from build123d import *

# Parameters (mm, degrees)
F1_DEPTH      = 40
F2_R          = 10
F3_DEPTH      = 180
F3_DEPTH_BACK = 20
F4_R          = 10
F5_DEPTH      = 20
F5_DEPTH_BACK = 180
F7_DEPTH      = 181.4
F9_DEPTH      = 244.2
F11_DEPTH     = 10
F12_R         = 2
F13_R         = 2


# Not quite as in the source:
# - a feature names something its author has since deleted; it is built from what else it names


with BuildPart() as f1:
    # F0 (on Top) → F1 (new body)
    with BuildSketch(Plane.XY):
        Polygon((-33.1370849898, -80), (33.1370849898, -80), (80, -33.1370849898), (80, 33.1370849898), (33.1370849898, 80), (-33.1370849898, 80), (-80, 33.1370849898), (-80, -33.1370849898), align=None)
        Polygon((60, -24.8528137424), (24.8528137424, -60), (-24.8528137424, -60), (-60, -24.8528137424), (-60, 24.8528137424), (-24.8528137424, 60), (24.8528137424, 60), (60, 24.8528137424), align=None, mode=Mode.SUBTRACT)
    extrude(amount=F1_DEPTH)

    # F2 (on face) → F3 (cut, two sides)
    with BuildSketch(Plane.XZ.offset(80)) as f3_sk:
        with Locations((0, 20)):
            Circle(F2_R)
    extrude(amount=-F3_DEPTH, mode=Mode.SUBTRACT)
    extrude(f3_sk.sketch, amount=F3_DEPTH_BACK, mode=Mode.SUBTRACT)

    # F4 (on face) → F5 (cut, two sides)
    with BuildSketch(Plane.YZ.offset(80)) as f5_sk:
        with Locations((0, 20)):
            Circle(F4_R)
    extrude(amount=F5_DEPTH, mode=Mode.SUBTRACT)
    extrude(f5_sk.sketch, amount=-F5_DEPTH_BACK, mode=Mode.SUBTRACT)

    # F6 (on face) → F7 (cut)
    with BuildSketch(Plane.XZ.offset(80)):
        Polygon((-33.1370849898, 40), (0, 40), (0, 51.6958795488), (-57.5, 51.6958795488), (-71.9271823764, 52.9654417948), (-71.9271823764, 40), (-57.5, 40), (-33.1370849898, 35.2627665258), align=None)
        with BuildLine():
            Line((0, 40), (0, 30))
            ThreePointArc((0, 30), (7.0710678119, 27.0710678119), (10, 20))
            Line((10, 20), (21.5, 20))
            Line((21.5, 20), (21.5, 33))
            Line((21.5, 33), (33.1370849898, 35.2627665258))
            Line((33.1370849898, 35.2627665258), (33.1370849898, 40))
            Line((33.1370849898, 40), (0, 40))
        make_face()
        Polygon((0, 51.6958795488), (0, 40), (33.1370849898, 40), (33.1370849898, 35.2627665258), (57.5, 40), (71.9271823764, 40), (71.9271823764, 52.9654417948), (57.5, 51.6958795488), align=None)
        with BuildLine():
            Line((-21.5, 20), (-10, 20))
            ThreePointArc((-10, 20), (-7.0710678119, 27.0710678119), (0, 30))
            Line((0, 30), (0, 40))
            Line((0, 40), (-33.1370849898, 40))
            Line((-33.1370849898, 40), (-33.1370849898, 35.2627665258))
            Line((-33.1370849898, 35.2627665258), (-21.5, 33))
            Line((-21.5, 33), (-21.5, 20))
        make_face()
    extrude(amount=-F7_DEPTH, mode=Mode.SUBTRACT)

    # F8 (on face) → F9 (cut)
    with BuildSketch(Plane.YZ.offset(80)):
        Polygon((33.1370849898, 0), (0, 0), (0, -11.1064584926), (57.5, -11.1064584926), (66.6687613726, -11.8878306821), (66.6687613726, 0), (57.5, 0), (33.1370849898, 4.7372334742), align=None)
        with BuildLine():
            ThreePointArc((10, 20), (7.0710678119, 12.9289321881), (0, 10))
            Line((0, 10), (0, 0))
            Line((0, 0), (33.1370849898, 0))
            Line((33.1370849898, 0), (33.1370849898, 4.7372334742))
            Line((33.1370849898, 4.7372334742), (21.5, 7))
            Line((21.5, 7), (21.5, 20))
            Line((21.5, 20), (10, 20))
        make_face()
        with BuildLine():
            ThreePointArc((0, 10), (-7.0710678119, 12.9289321881), (-10, 20))
            Line((-10, 20), (-21.5, 20))
            Line((-21.5, 20), (-21.5, 7))
            Line((-21.5, 7), (-33.1370849898, 4.7372334742))
            Line((-33.1370849898, 4.7372334742), (-33.1370849898, 0))
            Line((-33.1370849898, 0), (0, 0))
            Line((0, 0), (0, 10))
        make_face()
        Polygon((0, -11.1064584926), (0, 0), (-33.1370849898, 0), (-33.1370849898, 4.7372334742), (-57.5, 0), (-66.6687613726, 0), (-66.6687613726, -11.8878306821), (-57.5, -11.1064584926), align=None)
    extrude(amount=-F9_DEPTH, mode=Mode.SUBTRACT)

    # F10 (on face) → F11 (cut)
    with BuildSketch(Plane(origin=(56.5685424949, 56.5685424949, 0), x_dir=(-0.7071067812, 0.7071067812, 0), z_dir=(0.7071067812, 0.7071067812, 0))):
        with BuildLine():
            Line((-19.68193107, 12.9813232565), (1.7303785257, 10.0372808895))
            ThreePointArc((1.7303785257, 10.0372808895), (2.0021645777, 10.0093311061), (2.2752246058, 10))
            Line((2.2752246058, 10), (19.1370849898, 10))
            ThreePointArc((19.1370849898, 10), (21.9655121146, 11.1715728753), (23.1370849898, 14))
            Line((23.1370849898, 14), (23.1370849898, 23.055957633))
            ThreePointArc((23.1370849898, 23.055957633), (22.1519966238, 25.6847040718), (19.68193107, 27.0186767435))
            Line((19.68193107, 27.0186767435), (-1.7303785257, 29.9627191105))
            ThreePointArc((-1.7303785257, 29.9627191105), (-2.0021645777, 29.9906688939), (-2.2752246058, 30))
            Line((-2.2752246058, 30), (-19.1370849898, 30))
            ThreePointArc((-19.1370849898, 30), (-21.9655121146, 28.8284271247), (-23.1370849898, 26))
            Line((-23.1370849898, 26), (-23.1370849898, 16.944042367))
            ThreePointArc((-23.1370849898, 16.944042367), (-22.1519966238, 14.3152959282), (-19.68193107, 12.9813232565))
        make_face()
    extrude(amount=-F11_DEPTH, mode=Mode.SUBTRACT)

    # F12
    f12_edges = [f1.edges().sort_by_distance(p)[0] for p in [
        (33.137085, 65.857864, 18.527979),
        (33.965512, 65.029437, 11.171573),
        (41.92708, 57.067869, 10),
    ]]
    fillet(f12_edges, radius=F12_R)

    # F13
    f13_edges = [f1.edges().sort_by_distance(p)[0] for p in [
        (44.387085, 68.75, 0),
        (67.818542, 45.318542, 2.368617),
        (33.137085, 80, 17.631383),
        (45.318542, 67.818542, 37.631383),
        (80, 33.137085, 22.368617),
        (68.75, 44.387085, 40),
        (72.100505, 41.03658, 28.828427),
        (64.138937, 48.998148, 30),
        (57.984287, 55.152798, 29.990669),
        (50.22171, 62.915375, 28.490698),
        (40.904715, 72.23237, 25.684704),
        (40.208153, 72.928932, 18.527979),
        (41.03658, 72.100505, 11.171573),
        (48.998148, 64.138937, 10),
        (55.152798, 57.984287, 10.009331),
        (62.915375, 50.22171, 11.509302),
        (72.23237, 40.904715, 14.315296),
        (72.928932, 40.208153, 21.472021),
        (44.387085, -68.75, 0),
        (33.137085, -80, 17.631383),
        (45.318542, -67.818542, 37.631383),
        (68.75, -44.387085, 40),
        (80, -33.137085, 22.368617),
        (67.818542, -45.318542, 2.368617),
        (0, -80, 0),
        (27.318542, -80, 34.131383),
        (-44.387085, -68.75, 0),
        (-67.818542, -45.318542, 2.368617),
        (-80, -33.137085, 22.368617),
        (-68.75, -44.387085, 40),
        (-45.318542, -67.818542, 37.631383),
        (-33.137085, -80, 17.631383),
        (-44.387085, 68.75, 0),
        (-33.137085, 80, 17.631383),
        (-45.318542, 67.818542, 37.631383),
        (-68.75, 44.387085, 40),
        (-80, 33.137085, 22.368617),
        (-67.818542, 45.318542, 2.368617),
    ]]
    fillet(f13_edges, radius=F13_R)


solid = f1.part
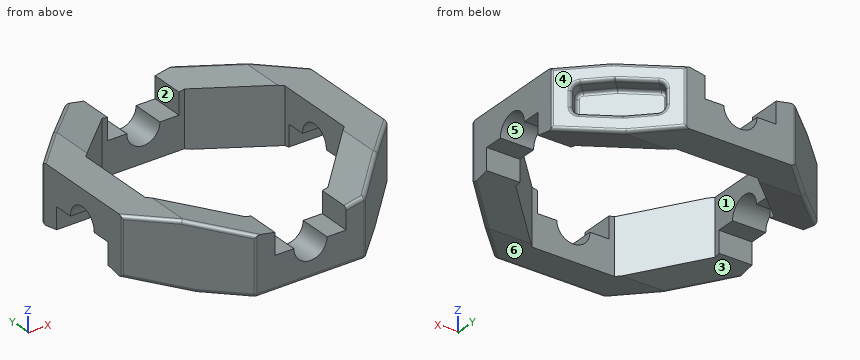
Input: part model. Units: mm. Frame: model coordinates. Face numbers are marked on the shaded views. A direction names the side the tool comes from. Round coordinates to 2 decimals unless told otherwise and drop trailing zeros. Write each loop counter-clockwise with the first axis right and the second up, starting at its lowest first coordinate (ties: lowest second). Pieces come first, ordered by that corner, then holes.
1) Ray query, L1, parallel to X at y = 36, z = 16.5; L2, parallel to Y at x = 22, z = 21. Return the intervals inside material, ascending.
2) Cut plane C-C (x = 0). Return the cut outline in (y, z).
3) Cut plane A-A (y = 0). Return the cut outline in (x, z).
4) Contact query for flat-ended pins moving along their axis: P1, Ø6.5, axis at x = 72, z = 10.5, coming from the -Y side; P2, Ø10.5, axis at y = 66, z = 25.5, coming from the +X side; P3, Ø6.5, axis at x = 69.5, z = 15.5, coming from the +Y side. Output: stop coordinate, or through.
5) Reachability of the marked faces 1, 2 and 3 from +Z, -Z, +X, -X, +Y, -Y: full face, straight path, thin tool, end or side. Return the list, or none.
6) Cut plane B-B (x = 16.5). Return the cut outline in (y, z).
7) Draft query along Y for the marked faces 4, 5 and 6. Return one class per face: pulls with the +Y half, pulls with the -Y half, needs draft (parallel to the pull), parting line crosses it, or undercut.
Geometry says:
1. L1: x = -77.14 to -48.85, 48.85 to 62.99, 68.69 to 77.14
1. L2: y = -80 to -60, 60 to 80
2. outline: (-80, 2) arc R2 ccw to (-78, 0) - (-60, 0) - (-60, 10) - (-80, 10) - close; (60, 0) - (80, 0) - (80, 10) - (60, 10) - close
3. outline: (-80, 30) - (-60, 30) - (-60, 40) - (-80, 40) - close; (60, 30) - (80, 30) - (80, 40) - (60, 40) - close
4. P1: stops at y = -44.39
4. P2: stops at x = 50.15
4. P3: stops at y = 43.33
5. face 1: +Z, -Z
5. face 2: +Z, +Y, -Y
5. face 3: -Z, +X, -X
6. outline: (-80, 2) arc R2 ccw to (-78, 0) - (-60, 0) - (-60, 20) - (-80, 20) - close; (60, 0) - (80, 0) - (80, 20) - (60, 20) - close
7. face 4: pulls with the +Y half
7. face 5: undercut
7. face 6: needs draft
